from build123d import *

# Parameters (mm, degrees)
SKETCH1_R           = 3.1
SKETCH1_R_2         = 2.5
BOSS_EXTRUDE1_DEPTH = 15
BOSS_EXTRUDE3_START = -5
SKETCH6_R           = 3.1
BOSS_EXTRUDE3_DEPTH = 5
BOSS_EXTRUDE4_DEPTH = 15
SKETCH8_R           = 2.6
CUT_EXTRUDE3_DEPTH  = 27
CUT_EXTRUDE4_DEPTH  = 89.777895192
SKETCH11_W          = 24
SKETCH11_H          = 0.25
BOSS_EXTRUDE5_DEPTH = 15
SKETCH12_W          = 24
SKETCH12_H          = 32
SKETCH12_H_2        = 23
BOSS_EXTRUDE6_DEPTH = 22
SKETCH13_R          = 6.1
CUT_EXTRUDE5_DEPTH  = 59.362710124
SKETCH14_W          = 24
SKETCH14_H          = 9
SKETCH14_R          = 1.2
BOSS_EXTRUDE7_DEPTH = 3
CHAMFER1_SIZE       = 2.5
CHAMFER2_SIZE       = 0.75


with BuildPart() as part:
    # Sketch1 → Boss-Extrude1 (new body)
    with BuildSketch(Plane.XY):
        with BuildLine():
            Line((-25.80048806, 37.524276553), (-49.80048806, 37.524276553))
            Line((-49.80048806, 37.524276553), (-49.80048806, -14.975723447))
            Line((-49.80048806, -14.975723447), (-41.80048806, -45.286414829))
            ThreePointArc((-41.80048806, -45.286414829), (-37.80048806, -49.286414829), (-33.80048806, -45.286414829))
            Line((-33.80048806, -45.286414829), (-25.80048806, -14.975723447))
            Line((-25.80048806, -14.975723447), (-25.80048806, 37.524276553))
        make_face()
        with Locations((-37.80048806, 25.524276553)):
            Circle(SKETCH1_R, mode=Mode.SUBTRACT)
        with Locations((-37.80048806, -2.975723447)):
            Circle(SKETCH1_R, mode=Mode.SUBTRACT)
        with Locations((-37.80048806, -45.286414829)):
            Circle(SKETCH1_R_2, mode=Mode.SUBTRACT)
    extrude(amount=BOSS_EXTRUDE1_DEPTH)

    # Sketch6 → Boss-Extrude3 (add)
    with BuildSketch(Plane.XY.offset(15).offset(BOSS_EXTRUDE3_START)):
        with Locations((-37.80048806, -2.975723447)):
            Circle(SKETCH6_R)
        with Locations((-37.80048806, 25.524276553)):
            Circle(SKETCH6_R)
    extrude(amount=BOSS_EXTRUDE3_DEPTH)

    # Sketch7 → Boss-Extrude4 (add)
    with BuildSketch(Plane.XY.offset(15)):
        Polygon((-51.800511672, 16.774276553), (-49.80048806, 16.774276553), (-49.80048806, -15.225723447), (-72.300511672, -15.225723447), (-72.300511672, 16.774276553), (-64.300511672, 16.774276553), (-64.300511672, -7.225723447), (-58.050499866, -7.225723447), (-51.800511672, -7.225723447), align=None)
    extrude(amount=-BOSS_EXTRUDE4_DEPTH)

    # Sketch8 → Cut-Extrude3 (cut)
    with BuildSketch(Plane.ZY.offset(72.300511672)):
        with Locations((7.5, 8.346782821)):
            Circle(SKETCH8_R)
    extrude(amount=-CUT_EXTRUDE3_DEPTH, mode=Mode.SUBTRACT)

    # Sketch10 → Cut-Extrude4 (cut, through all)
    with BuildSketch(Plane.XY.offset(15)):
        Polygon((-49.80048806, -15.225723447), (-49.80048806, -14.975723447), (-25.80048806, -14.975723447), (-25.80048806, -50.615055613), (-49.80048806, -50.615055613), align=None)
    extrude(amount=-CUT_EXTRUDE4_DEPTH, mode=Mode.SUBTRACT)

    # Sketch11 → Boss-Extrude5 (add)
    with BuildSketch(Plane.XY.offset(15)):
        with Locations((-37.80048806, -15.100723447)):
            Rectangle(SKETCH11_W, SKETCH11_H)
    extrude(amount=-BOSS_EXTRUDE5_DEPTH)

    # Sketch12 → Boss-Extrude6 (add)
    with BuildSketch(Plane.XY.offset(15)):
        with Locations((-37.80048806, 0.774276553)):
            Rectangle(SKETCH12_W, SKETCH12_H)
        with Locations((-37.80048806, -26.725723447)):
            Rectangle(SKETCH12_W, SKETCH12_H_2)
    extrude(amount=BOSS_EXTRUDE6_DEPTH)

    # Sketch13 → Cut-Extrude5 (cut, through all)
    with BuildSketch(Plane.ZY.offset(49.80048806)):
        with Locations(Location((26, 3.274276553, 0), (0, 0, 270))):
            Circle(SKETCH13_R)
        with Locations(Location((26, -24.725723447, 0), (0, 0, 270))):
            Circle(SKETCH13_R)
    extrude(amount=-CUT_EXTRUDE5_DEPTH, mode=Mode.SUBTRACT)

    # Sketch14 → Boss-Extrude7 (add)
    with BuildSketch(Plane(origin=(0, 37.524276553, 0), x_dir=(1, 0, 0), z_dir=(0, 1, 0))):
        with Locations((-37.80048806, 4.5)):
            Rectangle(SKETCH14_W, SKETCH14_H)
        with Locations(Location((-32.95048806, 2.9, 0), (0, 0, 270))):
            Circle(SKETCH14_R, mode=Mode.SUBTRACT)
        with Locations(Location((-42.55048806, 2.9, 0), (0, 0, 270))):
            Circle(SKETCH14_R, mode=Mode.SUBTRACT)
    extrude(amount=-BOSS_EXTRUDE7_DEPTH)

    # Chamfer1
    chamfer1_edges = [part.edges().sort_by_distance(p)[0] for p in [
        (-64.300511672, -7.225723447, 7.5),
        (-51.800511672, -7.225723447, 7.5),
    ]]
    chamfer(chamfer1_edges, length=CHAMFER1_SIZE)

    # Chamfer2
    chamfer2_edges = [part.edges().sort_by_distance(p)[0] for p in [
        (-37.80048806, 34.524276553, 0),
    ]]
    chamfer(chamfer2_edges, length=CHAMFER2_SIZE)


solid = part.part
Part model, mm, in its own coordinate system. A direction names the side the tool comes from. Coordinates: 2 decimals unless noted, no trailing zeros. Loops run counter-clockwise (first coordinate to the right, second up) from the corner with the lowest first, then second, coordinate; pieces in that order, holes last. Notation, with made-up numbers: M 60.25,81.25 L 76.25,81.25 A11 cw 76.25,101.25 Z; hole C 45,84.5 d1. An arc over 180 degrees is marked long. Use a Markdown table: item, result. Add a question column.
Q1. Cut at C-C (z = 7.5). Write the cut outline in (x, y).
Q2. Cut at B-B (y = 3). Write the cut outline in (x, z).
Q3. Cut at A-A (z = -2.9). Write the cut outline in (x, y).
Q4. Which spindle directions (+Z, -Z, +X, -X, +Y, -Y) get a long thin tool onto all of the face, cutting with end or side? Do faces 1 (the flat face through (-68, 16.774, 8)), 2 (the cylindrical face through (-68.36, 9.13, 9.98)), 3 (the cylindrical face through (-40.897, -2.839, 4.93)). Say none if no direction does.
Q5. Cut at D-D (x = -48.5). Write the cut outline in (y, z).
Q6. Pin check, flat tips, straight feed: P1, Ø7.5, axis at y = 9.5, z = 9, coming from the -X side; P2, Ø6, axis at x = -36.5, y = 22.5, coming from the +Z side; P3, Ø3, axis at x = -53, y = -10.5, coming from the -Z side; P4, Ø19.5, axis at y = 3.27, z = 26, coming from the -X side. Stop position of each tip, or through.
Q7. Probe L1, parallel to Z at x = -35, y = -25; L2, parallel to X at y = 35, z = -2; L3, parallel to Y at x = -35.5, z = 6. List the from-to ranges inside material, lowest first.
Q8. Mould opens along X. For faces 4 (the flat face through (-53.068, -5.993, 7.605)), 5 (the flat face through (-63.068, -5.958, 7.605)), 6 (the flat face through (-38, 37.524, 3)), 7 (the flat face through (-25.8, 0, 19)) say: +X half, -X half, draft (parallel to the pull), parting line (faces both ways), or undercut.
Worked out:
| question | item | result |
|---|---|---|
| 1 | outline | M -72.3,-15.23 L -25.8,-15.23 L -25.8,37.52 L -49.8,37.52 L -49.8,16.77 L -51.8,16.77 L -51.8,10.95 L -45.3,10.95 L -45.3,5.75 L -51.8,5.75 L -51.8,-4.73 L -54.3,-7.23 L -61.8,-7.23 L -64.3,-4.73 L -64.3,5.75 L -72.3,5.75 Z; M -72.3,10.95 L -64.3,10.95 L -64.3,16.77 L -72.3,16.77 Z; hole C -37.8,-2.98 d6.2; hole C -37.8,25.52 d6.2 |
| 2 | outline | M -72.3,0 L -64.3,0 L -64.3,15 L -72.3,15 Z; M -51.8,0 L -25.8,0 L -25.8,19.91 L -49.8,19.91 L -49.8,15 L -51.8,15 Z; M -49.8,32.09 L -25.8,32.09 L -25.8,37 L -49.8,37 Z |
| 3 | outline | M -49.8,34.52 L -43.75,34.52 L -43.75,37.52 L -49.8,37.52 Z; M -41.35,34.52 L -34.15,34.52 L -34.15,37.52 L -41.35,37.52 Z; M -31.75,34.52 L -25.8,34.52 L -25.8,37.52 L -31.75,37.52 Z |
| 4 | face 1 | +Z, -Z, -X, +Y |
| 4 | face 2 | -X |
| 4 | face 3 | -Z |
| 5 | outline | M -38.23,15 L -15.23,15 L -15.23,0 L 33.77,0 L 34.52,-0.75 L 34.52,-9 L 37.52,-9 L 37.52,15 L 16.77,15 L 16.77,37 L -38.23,37 Z; hole C -24.73,26 d12.2; hole C 3.27,26 d12.2; hole C 8.35,7.5 d5.2 |
| 6 | P1 | stops at x = -72.3 |
| 6 | P2 | stops at z = 15 |
| 6 | P3 | stops at z = 0 |
| 6 | P4 | stops at x = -49.8 |
| 7 | L1 | z = 15 to 19.91, 32.09 to 37 |
| 7 | L2 | x = -49.8 to -43.34, -41.76 to -33.74, -32.16 to -25.8 |
| 7 | L3 | y = -15.23 to -5.05, -0.9 to 23.45, 27.6 to 37.52 |
| 8 | face 4 | undercut |
| 8 | face 5 | undercut |
| 8 | face 6 | draft |
| 8 | face 7 | +X half |
